Autodesk Inventor part; units mm, degrees
ref_plane "YZ Plane" through (0, 0, 0) normal (1, 0, 0) x (0, 1, 0)
ref_plane "XY Plane" through (0, 0, 0) normal (0, 0, 1) x (1, 0, 0)
sketch "Sketch2" plane through (0, 0, 0) normal (1, 0, 0) x (0, 1, 0)
  circle A0 centre (27, 120) radius 7.5
  line L0 (27, 120) -> (34.5, 120)
  point P0 (0, 0)
ref_plane "Work Plane1" through (0, 34.5, 120) normal (0, 1, 0) x (-1, 0, 0)
sketch "Sketch3" plane through (0, 34.5, 120) normal (0, 1, 0) x (-1, 0, 0)
  line L0 (0, -120) -> (0, 59.5473) construction
  line L1 (-25, 10) -> (25, 10)
  line L2 (25, 10) -> (25, -10)
  line L3 (25, -10) -> (-25, -10)
  line L4 (-25, -10) -> (-25, 10)
  line L5 (-25, 0) -> (25, 0) construction
  point P0 (0, 0)
  point P1 (0, 0)
  point P2 (0, 0)
  dimension "d2" = 20
  dimension "d3" = 50
extrude "Extrusion1" add sketch "Sketch3" along normal blind 1
sketch "Sketch4" plane through (0, 35.5, 120) normal (0, 1, 0) x (1, 0, 0)
  line L0 (25, -10) -> (25, 10) construction
  line L1 (25, 0) -> (-25, 0) construction
  line L2 (-25, 10) -> (-25, -10) construction
  line L3 (-25, -10) -> (25, -10) construction
  line L4 (20, -10) -> (20, 10) construction
  line L5 (25, 10) -> (-25, 10) construction
  line L6 (-20, -10) -> (-20, 10) construction
  point P0 (0, 120)
  point P1 (20, 0)
  point P2 (-20, 0)
  dimension "d6" = 5
  dimension "d7" = 5
hole "Hole1" at (20, 35.5, 120) at (-20, 35.5, 120) direction (0, -1, 0) diameter 4.1 end through all
fillet "Fillet1" radius 2 4 edges at (25, 35, 130) (25, 35, 110) (-25, 35, 130) (-25, 35, 110)
ref_plane "Work Plane2" through (-23, 34.5, 120) normal (0, 0, 1) x (1, 0, 0)
properties part number "Plate" material "Steel, High Strength, Low Alloy"
Check sheet for the modelled part. Datum: model origin and axes. Units: mm. Give positions to 0.01 mm unless a question says otherwise; leave off trailing zeros. Order: outer loops, then holes, each group sorted by start corner. A loop starts at its lowest first (then second) coordinate and runs counter-clockwise, first axis right, second up. Notation, with made-up numbers: M -14.75,71.5 L 8.25,71.5 A20 cw 8.25,77.5 Z; hole C 0.5,50 d1. An arc over 180 degrees is marked long. Answer in a Markdown table with one row per item. Add a question column.
Q1. Gauge pin test, flat end, axial feed: pin 1 Ø2.5 at (x, z) = (20, 120) entering from +Y. Record the tip position at first contact, or that the pin passes through.
Q2. Sectioned sample at B-B, the plane x = -20. Record the boundary of the cut face in (y, z).
Q3. Release check for a two-part mould opening along X. For faces 1 (the cylindrical face through (24.43, 35.01, 110.6)), 2 (the flat face through (0, 34.5, 120)), 3 (the cylindrical face through (-20.616, 34.993, 121.955)), 4 (the cylindrical face through (19.384, 34.993, 121.955)) record: released by +X, released by -X, zero draft, split by the parting line, or undercut.
Q4. Sectioned sample at A-A, the plane y = 34.8. Record the boundary of the cut face in (x, z).
Q5. Thickness scan on L1, parallel to X at y = 35.2, z = 120; L2, parallel to Z at x = 20, y = 35.1. Record the ranges inside material, lowest first.
Q6. Sectioned sample at C-C, the plane z = 120. Record the boundary of the cut face in (x, y), and give its area (3 significant figures).
Verdict:
| question | item | result |
|---|---|---|
| 1 | pin 1 | through |
| 2 | outline | M 34.5,110 L 35.5,110 L 35.5,117.95 L 34.5,117.95 Z; M 34.5,122.05 L 35.5,122.05 L 35.5,130 L 34.5,130 Z |
| 3 | face 1 | released by +X |
| 3 | face 2 | zero draft |
| 3 | face 3 | undercut |
| 3 | face 4 | undercut |
| 4 | outline | M -25,112 A2 ccw -23,110 L 23,110 A2 ccw 25,112 L 25,128 A2 ccw 23,130 L -23,130 A2 ccw -25,128 Z; hole C -20,120 d4.1; hole C 20,120 d4.1 |
| 5 | L1 | -25 to -22.05, -17.95 to 17.95, 22.05 to 25 |
| 5 | L2 | 110 to 117.95, 122.05 to 130 |
| 6 | outline | M -25,34.5 L -22.05,34.5 L -22.05,35.5 L -25,35.5 Z; M -17.95,34.5 L 17.95,34.5 L 17.95,35.5 L -17.95,35.5 Z; M 22.05,34.5 L 25,34.5 L 25,35.5 L 22.05,35.5 Z |
| 6 | area | 41.8 mm² |
